Autodesk Inventor part; units mm, degrees
ref_plane "YZ Plane" through (0, 0, 0) normal (1, 0, 0) x (0, 1, 0)
ref_plane "XZ Plane" through (0, 0, 0) normal (0, 1, 0) x (-1, 0, 0)
ref_plane "XY Plane" through (0, 0, 0) normal (0, 0, 1) x (1, 0, 0)
sketch "Sketch1" plane through (0, 0, 0) normal (0, 1, 0) x (-1, 0, 0)
  line L0 (40, 50) -> (-40, 50)
  line L1 (-40, 50) -> (-40, -50)
  line L2 (-40, -50) -> (40, -50)
  line L3 (40, -50) -> (40, 50)
  line L4 (40, 50) -> (-40, -50) construction
  line L5 (-40, 50) -> (40, -50) construction
  point P0 (0, 0)
  dimension "d0" = 80
  dimension "d1" = 100
extrude "Extrusion1" add sketch "Sketch1" along normal blind 3
sketch "Sketch2" plane through (0, 3, 0) normal (0, 1, 0) x (1, 0, 0)
  line L0 (-40, 50) -> (-40, -50)
  line L1 (40, -50) -> (40, 50)
  line L2 (-40, -50) -> (40, -50)
  line L3 (40, -50) -> (40, -47)
  line L4 (40, -47) -> (-40, -47)
  line L5 (-40, -47) -> (-40, -50)
  point P0 (0, 0)
  dimension "d4" = 3
extrude "Extrusion2" add sketch "Sketch2" along normal blind 85
sketch "Sketch4" plane through (40, 3, 47) normal (0, 0, -1) x (-1, 0, 0)
  circle A0 centre (40, 45) radius 22.5
  line L0 (0, 0) -> (80, 0)
  line L1 (0, 0) -> (0, 85)
  circle A1 centre (12.5, 45) radius 1.5
  circle A2 centre (40, 72.5) radius 1.5
  circle A3 centre (67.5, 45) radius 1.5
  circle A4 centre (40, 17.5) radius 1.5
  line L2 (0, 85) -> (80, 85)
  point P0 (40, -3)
  dimension "d7" = 45
  dimension "d9" = 40
  dimension "d10" = 3
  dimension "d11" = 3
  dimension "d12" = 3
  dimension "d13" = 3
  dimension "d14" = 27.5
  dimension "d15" = 27.5
  dimension "d16" = 27.5
  dimension "d17" = 27.5
  dimension "d21" = 40
extrude "Extrusion3" cut sketch "Sketch4" against normal blind 3
fillet "Fillet1" radius 40 2 edges at (40, 88, 48.5) (-40, 88, 48.5)
fillet "Fillet2" radius 5 1 edges at (0, 3, 47)
fillet "Fillet3" radius 7.5 1 edges at (0, 0, 50)
fillet "Fillet4" radius 10 2 edges at (40, 1.5, -50) (-40, 1.5, -50)
sketch "Sketch7" plane through (0, 3, 0) normal (0, 1, 0) x (1, 0, 0)
  circle A0 centre (28, -20) radius 2.5
  circle A1 centre (28, 25) radius 2.5
  circle A2 centre (-28, 25) radius 2.5
  circle A3 centre (-28, -20) radius 2.5
  line L0 (40, -42) -> (40, 40)
  line L1 (30, 50) -> (-30, 50)
  line L2 (-40, 40) -> (-40, -42)
  line L3 (15, -30) -> (-15, -30)
  line L4 (-15, -30) -> (-15, 30)
  line L5 (-15, 30) -> (15, 30)
  line L6 (15, 30) -> (15, -30)
  line L7 (15, -30) -> (-15, 30) construction
  line L8 (-15, -30) -> (15, 30) construction
  point P0 (0, 0)
  dimension "d25" = 5
  dimension "d26" = 5
  dimension "d27" = 5
  dimension "d28" = 5
  dimension "d29" = 12
  dimension "d30" = 70
  dimension "d31" = 25
  dimension "d32" = 12
  dimension "d33" = 70
  dimension "d34" = 25
  dimension "d35" = 30
  dimension "d36" = 60
extrude "Extrusion4" cut sketch "Sketch7" against normal blind 85
fillet "Fillet5" radius 10 4 edges at (-15, 1.5, 30) (15, 1.5, 30) (15, 1.5, -30) (-15, 1.5, -30)
properties part number "Holder Water Pump"
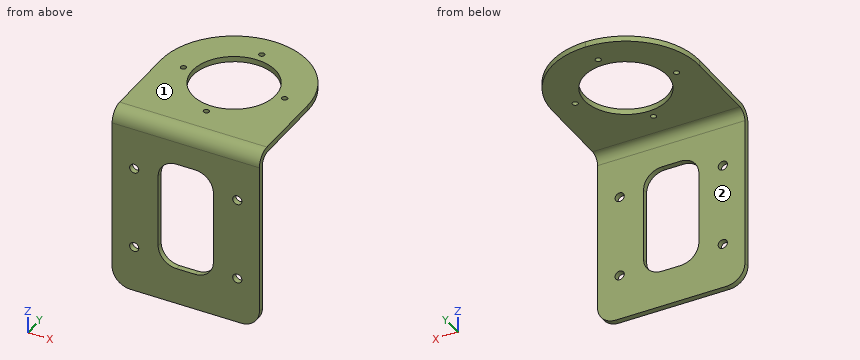
The model under review builds one solid part; all positions refer to its coordinate system, in mm. Face numbers are marked on the shaded views. A direction names the side the tool comes from. Round coordinates to 2 decimals unless told otherwise and drop trailing zeros. Loops run counter-clockwise (first coordinate to the right, second up) from the corner with the lowest first, then second, coordinate; pieces in that order, holes last. Notation, with made-up numbers: (-38, 47) -> (-16, 47) arc R9 ccw to (-16, 58) -> close; hole circle Ø5 at (-14.5, 41). An arc over 180 degrees is marked (long way). Return JSON: item names as keys, results as strings.
(1) For line 1 (X direction, y = 1, z = 20); line 2 (Z direction, x = -28, y = 1.6); line 3 (X direction, y = 1.85, z = -25), list the stretches that pass through material, from the lowest coordinate up.
Solved:
{"line 1": "-40 to -30.5, -25.5 to -15, 15 to 25.5, 30.5 to 40", "line 2": "-50 to -27.5, -22.5 to 17.5, 22.5 to 47.13", "line 3": "-40 to -30.5, -25.5 to -13.66, 13.66 to 25.5, 30.5 to 40"}
(2) For the marked faces 1 and 2, list the 3-axis set-ups (+Z, -Z, +X, -X, +Y, -Y) from which the entire face can be reached by the end or side of a thin tool; tool diameter is ignored.
Solved:
{"face 1": "+Z, +X, -X, +Y, -Y", "face 2": "-Z, +X, -X, +Y"}
(3) Add section D-D on x = 27.5. Write out the cut boundary in (y, z), plus the area to 3 significant figures.
Solved:
{"outline": "(0, -50) -> (3, -50) -> (3, -27.45) -> (0, -27.45) -> close; (0, -22.55) -> (3, -22.55) -> (3, 17.55) -> (0, 17.55) -> close; (0, 22.45) -> (3, 22.45) -> (3, 42) arc R5 cw to (8, 47) -> (46.5, 47) -> (46.5, 50) -> (7.5, 50) arc R7.5 ccw to (0, 42.5) -> close; (49.5, 47) -> (77.05, 47) -> (77.05, 50) -> (49.5, 50) -> close", "area": "477 mm2"}
(4) Add section C-C on x = -3.5. Write out the cut boundary in (y, z), plus the area to 3 significant figures.
Solved:
{"outline": "(0, -50) -> (3, -50) -> (3, -30) -> (0, -30) -> close; (0, 30) -> (3, 30) -> (3, 42) arc R5 cw to (8, 47) -> (25.77, 47) -> (25.77, 50) -> (7.5, 50) arc R7.5 ccw to (0, 42.5) -> close; (70.23, 47) -> (87.85, 47) -> (87.85, 50) -> (70.23, 50) -> close", "area": "234 mm2"}
(5) Add section B-B on y = 75.5. Write out the cut boundary in (x, z), plus the area to 3 significant figures.
Solved:
{"outline": "(-29.05, 47) -> (-1.5, 47) -> (-1.5, 50) -> (-29.05, 50) -> close; (1.5, 47) -> (29.05, 47) -> (29.05, 50) -> (1.5, 50) -> close", "area": "165 mm2"}
(6) For pin 1 (2.5 mm diameter, centred on x = -2, y = 1.5, fed in from +Z), flat-tipped, find the tip position at first contact; note if it passes through.
Solved:
{"pin 1": "z = 48.3"}
(7) Add section A-A on z = -16. Write out the cut boundary in (x, y).
Solved:
{"outline": "(-40, 0) -> (-15, 0) -> (-15, 3) -> (-40, 3) -> close; (15, 0) -> (40, 0) -> (40, 3) -> (15, 3) -> close"}
